Design review of the part built by this model. Coordinates are the model's own, in mm. Round coordinates to 2 decimals unless told otherwise and drop trailing zeros. Order: outer loops, then holes, each group sorted by start corner. A loop starts at its lowest first (then second) coordinate and runs counter-clockwise, first axis right, second up. Notation, with made-up numbers: (-7.75, 60.5) - (50.25, 60.5) arc R23 cw to (50.25, 69.5) - close; hole circle Ø6 at (77, 46). An arc over 180 degrees is marked (long way). Write item = value, one per line.
from build123d import *

# Parameters (mm, degrees)
F1_DEPTH = 12
F2_R     = 0.5
F3_DEPTH = 1


with BuildPart() as f1:
    # F0 (on Top) → F1 (new body)
    with BuildSketch(Plane.XY):
        Polygon((126.98753, -74.492732), (1.018833, 147.220793), (-128.006364, -72.728061), align=None)
    extrude(amount=F1_DEPTH)

    # F2 (on face) → F3 (join)
    with BuildSketch(Plane.XY.offset(12)):
        Circle(F2_R)
    extrude(amount=F3_DEPTH)


solid = f1.part
Item 1: Take a section at A-A, the plane y = 42. State the section outline as (x, z) points.
Data:
outline = (-60.71, 0) - (60.8, 0) - (60.8, 12) - (-60.71, 12) - close
Item 2: Take a section at C-C, the plane z = 9.25. State the section outline as (x, y) points.
Data:
outline = (-128.01, -72.73) - (126.99, -74.49) - (1.02, 147.22) - close
Item 3: Take a section at B-B, the plane x = 88. State the section outline as (y, z) points.
Data:
outline = (-74.22, 0) - (-5.87, 0) - (-5.87, 12) - (-74.22, 12) - close
Item 4: For line 1 along Z through (x, y) = (68, -42); line 2 along X through (y, z) = (61, 9.5); line 3 along Y through (x, z) = (-63.5, 7), list the stretches that pass through material, from the lowest coordinate up. Write a range as [from, to].
Data:
line_1 = [0, 12]
line_2 = [-49.56, 50.01]
line_3 = [-73.17, 37.24]
Item 5: Insertion check: P1, Ø6, axis at y = 21, z = 11, coming from the -X side; P2, Ø1, axis at x = -71, z = 5, coming from the -Y side; P3, Ø4, axis at y = 5, z = 11, coming from the +X side. Each pin has a flat end and moves straight along its axis. Give the tip position at first contact, or say it passes through.
Data:
P1 = -74.78
P2 = -73.13
P3 = 82.96
